Here's the drawing with two shaded views (mm, measured from the low corner). I have some questions. A direction names the side the tool comes from. Give positions to 0.01 mm unless a question says otherwise; leave off trailing zeros. Loops run counter-clockwise (first coordinate to the right, second up) from the corner with the lowest first, then second, coordinate; pieces in that order, holes last. Notation, with made-up numbers: (87, 1.25) - (138, 1.25) arc R26 cw to (138, 27.25) - close; hole circle Ø11 at (-39, 14). An arc over 180 degrees is marked (long way). Use a Markdown table: item, result. Add a question column.
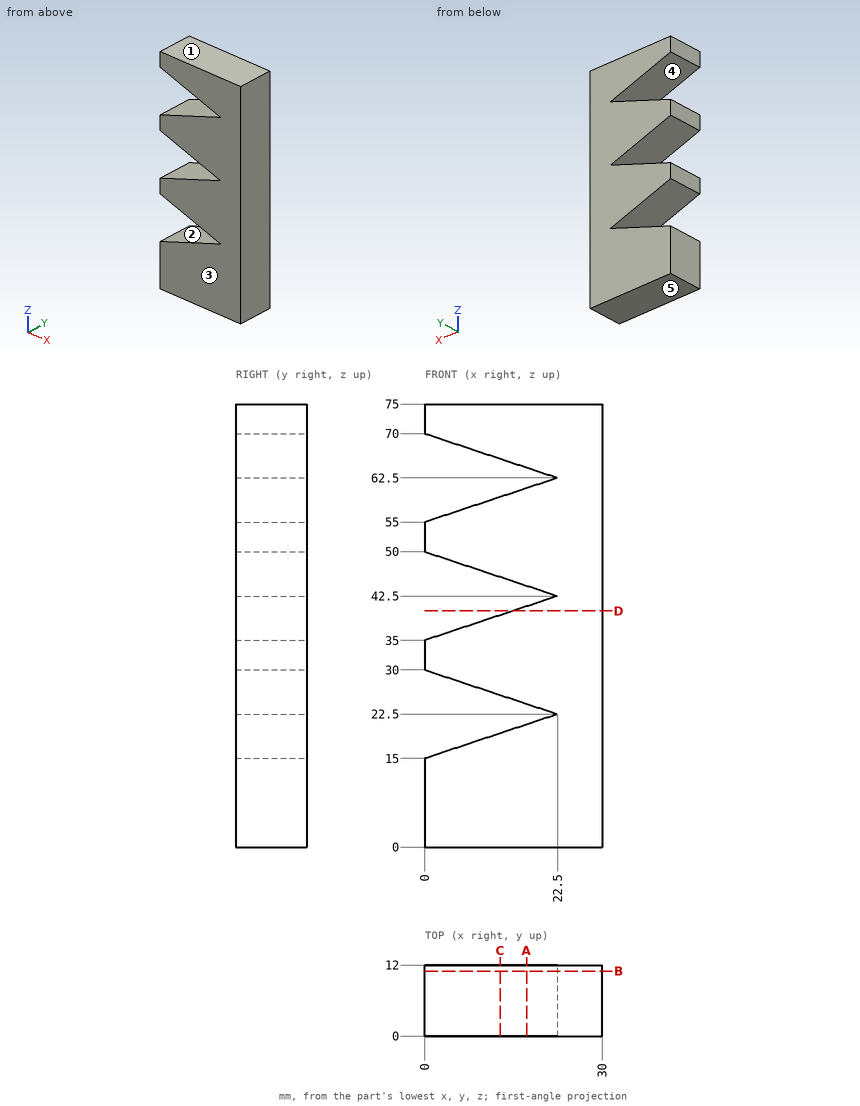
1. Suppose I cut it at A-A (x = 17.25). List the corners of the cut face in (y, z) for me.
2. Suppose I cut it at C-C (x = 12.75). List the corners of the cut face in (y, z) for me.
3. Suppose I cut it at D-D (z = 40). List the corners of the cut face in (x, y) for me.
4. Please list where these lines run through material, in increasing order: line 1 along Z through (x, y) = (19, 6); line 2 along Z through (x, y) = (12.5, 10). Write a range as [from, to].
5. Suppose I cut it at B-B (y = 11). List the corners of the cut face in (x, z) for me.
6. Will this pin go through, and if not, where does the flat tip stop? P1, Ø4, axis at x = 20.5, z = 55, coming from the -Y side.
7. If we mould it in two halves opening along Z, with no side actions, what happens to the marked faces 3, 4 and 5? For each: released by +Z, released by -Z, zero draft, split by the parting line, or undercut.
8. On a 3-axis mill with a long thin cutter (end or side, diameter ignored), from which of +Z, -Z, +X, -X, +Y, -Y can I reach the whole of each face in a straight line? I mean the marked faces 1 and 2. Say none if no direction works.
Results below:
| question | item | result |
|---|---|---|
| 1 | outline | (0, 0) - (12, 0) - (12, 20.75) - (0, 20.75) - close; (0, 24.25) - (12, 24.25) - (12, 40.75) - (0, 40.75) - close; (0, 44.25) - (12, 44.25) - (12, 60.75) - (0, 60.75) - close; (0, 64.25) - (12, 64.25) - (12, 75) - (0, 75) - close |
| 2 | outline | (0, 0) - (12, 0) - (12, 19.25) - (0, 19.25) - close; (0, 25.75) - (12, 25.75) - (12, 39.25) - (0, 39.25) - close; (0, 45.75) - (12, 45.75) - (12, 59.25) - (0, 59.25) - close; (0, 65.75) - (12, 65.75) - (12, 75) - (0, 75) - close |
| 3 | outline | (15, 0) - (30, 0) - (30, 12) - (15, 12) - close |
| 4 | line 1 | [0, 21.33], [23.67, 41.33], [43.67, 61.33], [63.67, 75] |
| 4 | line 2 | [0, 19.17], [25.83, 39.17], [45.83, 59.17], [65.83, 75] |
| 5 | outline | (0, 0) - (30, 0) - (30, 75) - (0, 75) - (0, 70) - (22.5, 62.5) - (0, 55) - (0, 50) - (22.5, 42.5) - (0, 35) - (0, 30) - (22.5, 22.5) - (0, 15) - close |
| 6 | P1 | y = 0 |
| 7 | face 3 | zero draft |
| 7 | face 4 | undercut |
| 7 | face 5 | released by -Z |
| 8 | face 1 | +Z, +X, -X, +Y, -Y |
| 8 | face 2 | -X, +Y, -Y |
